Can you work these out from the model? Positions are in its coordinate system, mm. Face numbers are marked on the shaded views. Round coordinates to 2 decimals unless told otherwise and drop trailing zeros. Order: outer loops, then holes, each group sorted by start corner. A loop starts at its lowest first (then second) coordinate and runs counter-clockwise, first axis right, second up. Notation, with made-up numbers: (-1, -38) -> (32, -38) arc R16 ccw to (32, -13) -> close; hole circle Ø6 at (19, 26.25). An arc over 180 degrees is marked (long way). One line per item, written item: value.
```python
from build123d import *

# Parameters (mm, degrees)
SKETCH1_R           = 15
SKETCH1_R_2         = 10
BOSS_EXTRUDE1_DEPTH = 150
SKETCH2_W           = 35
SKETCH2_H           = 35
BOSS_EXTRUDE2_DEPTH = 5
CUT_EXTRUDE5_DEPTH  = 20
BOSS_EXTRUDE4_START = 10
SKETCH12_R          = 15
BOSS_EXTRUDE4_DEPTH = 10
SKETCH13_R          = 5
BOSS_EXTRUDE5_DEPTH = 10
CUT_EXTRUDE6_START  = 20
CUT_EXTRUDE6_DEPTH  = 20
SKETCH15_R          = 4.05
BOSS_EXTRUDE6_DEPTH = 7
SKETCH16_R          = 2.9
BOSS_EXTRUDE7_DEPTH = 35
SKETCH17_W          = 8
SKETCH17_H          = 27.5
SKETCH17_H_2        = 7.5
SKETCH17_W_2        = 7
CUT_EXTRUDE7_DEPTH  = 184.674984688
CUT_EXTRUDE11_DEPTH = 50
CUT_EXTRUDE13_START = 3
CUT_EXTRUDE13_DEPTH = 3


with BuildPart() as part:
    # Sketch1 → Boss-Extrude1 (new body)
    with BuildSketch(Plane.XY):
        Circle(SKETCH1_R)
        Circle(SKETCH1_R_2, mode=Mode.SUBTRACT)
    extrude(amount=BOSS_EXTRUDE1_DEPTH)

    # Sketch2 → Boss-Extrude2 (add)
    with BuildSketch(Plane.XY.offset(150)):
        Rectangle(SKETCH2_W, SKETCH2_H)
    extrude(amount=BOSS_EXTRUDE2_DEPTH)

    # Sketch10 → Cut-Extrude5 (cut)
    with BuildSketch(Plane(origin=(0, 0, 0), x_dir=(-1, 0, 0), z_dir=(0, 0, -1))):
        with BuildLine():
            Line((10, 0), (15, 0))
            ThreePointArc((15, 0), (0, 15), (-15, 0))
            Line((-15, 0), (-10, 0))
            ThreePointArc((-10, 0), (0, 10), (10, 0))
        make_face()
    extrude(amount=-CUT_EXTRUDE5_DEPTH, mode=Mode.SUBTRACT)

    # Sketch12 → Boss-Extrude4 (add)
    with BuildSketch(Plane(origin=(0, 0, 0), x_dir=(-1, 0, 0), z_dir=(0, 0, -1)).offset(BOSS_EXTRUDE4_START)):
        Circle(SKETCH12_R)
    extrude(amount=-BOSS_EXTRUDE4_DEPTH)

    # Sketch13 → Boss-Extrude5 (add)
    with BuildSketch(Plane(origin=(0, 0, -10), x_dir=(-1, 0, 0), z_dir=(0, 0, -1))):
        Circle(SKETCH13_R)
    extrude(amount=BOSS_EXTRUDE5_DEPTH)

    # Sketch14 → Cut-Extrude6 (cut)
    with BuildSketch(Plane(origin=(0, 0, 150), x_dir=(-1, 0, 0), z_dir=(0, 0, -1)).offset(CUT_EXTRUDE6_START)):
        with BuildLine():
            Line((-10.606601718, 10.606601718), (-7.071067812, 7.071067812))
            ThreePointArc((-7.071067812, 7.071067812), (0, 10), (7.071067812, 7.071067812))
            Line((7.071067812, 7.071067812), (10.606601718, 10.606601718))
            ThreePointArc((10.606601718, 10.606601718), (0, 15), (-10.606601718, 10.606601718))
        make_face()
    extrude(amount=-CUT_EXTRUDE6_DEPTH, mode=Mode.SUBTRACT)

    # Sketch15 → Boss-Extrude6 (add)
    with BuildSketch(Plane(origin=(0, 0, -20), x_dir=(-1, 0, 0), z_dir=(0, 0, -1))):
        Circle(SKETCH15_R)
    extrude(amount=BOSS_EXTRUDE6_DEPTH)

    # Sketch16 → Boss-Extrude7 (add)
    with BuildSketch(Plane.ZY.offset(17.5)):
        with BuildLine():
            Line((155, 10), (165, 10))
            ThreePointArc((165, 10), (175, 0), (165, -10))
            Line((165, -10), (155, -10))
            Line((155, -10), (155, 10))
        make_face()
        with Locations((165, 0)):
            Circle(SKETCH16_R, mode=Mode.SUBTRACT)
    extrude(amount=-BOSS_EXTRUDE7_DEPTH)

    # Sketch17 → Cut-Extrude7 (cut, through all)
    with BuildSketch(Plane.XY.offset(155)):
        with Locations((-13.5, -3.75)):
            Rectangle(SKETCH17_W, SKETCH17_H)
        with Locations((-13.5, 13.75)):
            Rectangle(SKETCH17_W, SKETCH17_H_2)
        with Locations((0, 13.75)):
            Rectangle(SKETCH17_W_2, SKETCH17_H_2)
        with Locations((0, -3.75)):
            Rectangle(SKETCH17_W_2, SKETCH17_H)
        with Locations((13.5, 13.75)):
            Rectangle(SKETCH17_W, SKETCH17_H_2)
        with Locations((13.5, -3.75)):
            Rectangle(SKETCH17_W, SKETCH17_H)
    extrude(amount=CUT_EXTRUDE7_DEPTH, mode=Mode.SUBTRACT)

    # Sketch20 → Cut-Extrude11 (cut)
    with BuildSketch(Plane(origin=(0, 0, -10), x_dir=(-1, 0, 0), z_dir=(0, 0, -1))):
        with BuildLine():
            ThreePointArc((1.5, -13.416407865), (0.751163705, -13.479085766), (0, -13.5))
            Line((0, -13.5), (0, -15))
            ThreePointArc((0, -15), (0.750941626, -14.981191097), (1.5, -14.924811557))
            Line((1.5, -14.924811557), (1.5, -13.416407865))
        make_face()
        with BuildLine():
            ThreePointArc((0, -13.5), (-0.751163705, -13.479085766), (-1.5, -13.416407865))
            Line((-1.5, -13.416407865), (-1.5, -14.924811557))
            ThreePointArc((-1.5, -14.924811557), (-0.750941626, -14.981191097), (0, -15))
            Line((0, -15), (0, -13.5))
        make_face()
    extrude(amount=-CUT_EXTRUDE11_DEPTH, mode=Mode.SUBTRACT)

    # Sketch23 → Cut-Extrude13 (cut)
    with BuildSketch(Plane(origin=(0, 0, 40), x_dir=(-1, 0, 0), z_dir=(0, 0, -1)).offset(CUT_EXTRUDE13_START)):
        with BuildLine():
            Line((-1.5, -14.924811557), (-1.5, -13.416407865))
            ThreePointArc((-1.5, -13.416407865), (-4.76963682, -12.629353293), (-7.743281891, -11.058552598))
            Line((-7.743281891, -11.058552598), (-8.603646545, -12.287280664))
            ThreePointArc((-8.603646545, -12.287280664), (-5.221116804, -14.062003389), (-1.5, -14.924811557))
        make_face()
    extrude(amount=-CUT_EXTRUDE13_DEPTH, mode=Mode.SUBTRACT)


solid = part.part
```
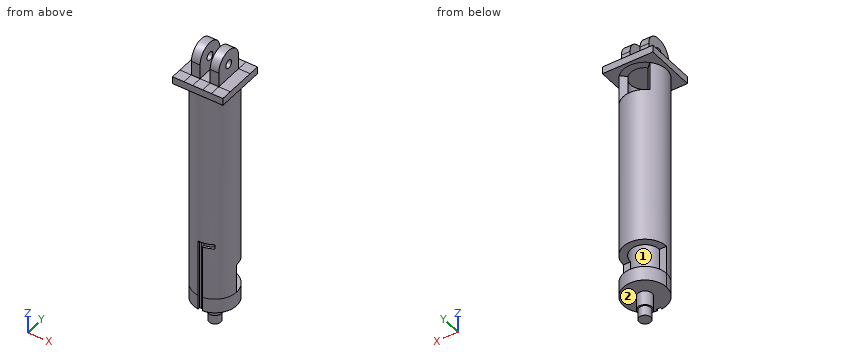
Q1. We'd pull the mould along Z, two halves only. Please class the marked faces 1 and 2: released by +Z, released by -Z, zero draft, split by the parting line, or undercut.
Answers below:
face 1: undercut
face 2: released by -Z
Q2. I want a section at C-C on z = 134.5. List the corners of the cut face in (x, y) for me, plus the area to 3 significant figures.
Answers below:
outline: (-10.61, 10.61) arc R15 ccw (long way) to (10.61, 10.61) -> (7.07, 7.07) arc R10 cw (long way) to (-7.07, 7.07) -> close
area: 295 mm^2
Q3. I want a section at A-A on y = -7. List the corners of the cut face in (x, z) for me.
Answers below:
outline: (-17.5, 150) -> (-13.27, 150) -> (-13.27, -10) -> (13.27, -10) -> (13.27, 150) -> (17.5, 150) -> (17.5, 155) -> (9.5, 155) -> (9.5, 172.14) -> (3.5, 172.14) -> (3.5, 155) -> (-3.5, 155) -> (-3.5, 172.14) -> (-9.5, 172.14) -> (-9.5, 155) -> (-17.5, 155) -> close; hole (-7.14, 0) -> (7.14, 0) -> (7.14, 150) -> (-7.14, 150) -> close
Q4. I want a section at B-B on z = 98.5. List the corners of the cut face in (x, y) for me, plus the area to 3 significant figures.
Answers below:
outline: circle Ø30 at (0, 0); hole circle Ø20 at (0, 0)
area: 393 mm^2
Q5. Please list where these lines run through material, in increasing order: line 1 along Z through (x, y) = (-2, 13.5); line 2 along Y through (x, z) = (7.85, 165); line 3 along X through (y, z) = (0, 115).
Answers below:
line 1: -10 to 0, 20 to 130, 150 to 155
line 2: -10 to -2.9, 2.9 to 10
line 3: -15 to -10, 10 to 15
Q6. Will these pins go through, and if not, where does the flat tip stop? pin 1 Ø5.5 at (x, y) = (-0.5, -13.5) entering from +Z; pin 2 Ø10 at (x, y) = (13, 9) entering from +Z; pin 3 Ø8 at (x, z) = (-9.5, 15.5) entering from +Y.
Answers below:
pin 1: z = 155
pin 2: z = 173.4
pin 3: y = 0
